Geometry check sheet. Reference: drawing and pictorial views, mm from the part's lowest x, y, z. Give positions to 0.01 mm unless a question says otherwise; leave off trailing zeros. Write each loop counter-clockwise with the first axis right and the second up, starting at its lowest first coordinate (ties: lowest second). Pieces come first, ordered by that corner, then holes. Notation, with made-up numbers: (-14.75, 6.25) -> (25.25, 6.25) arc R21 cw to (25.25, 40.25) -> close; hole circle Ø2 at (-24, 80.25). An arc over 180 degrees is marked (long way). Use a Markdown table: item, result. Add a question column.
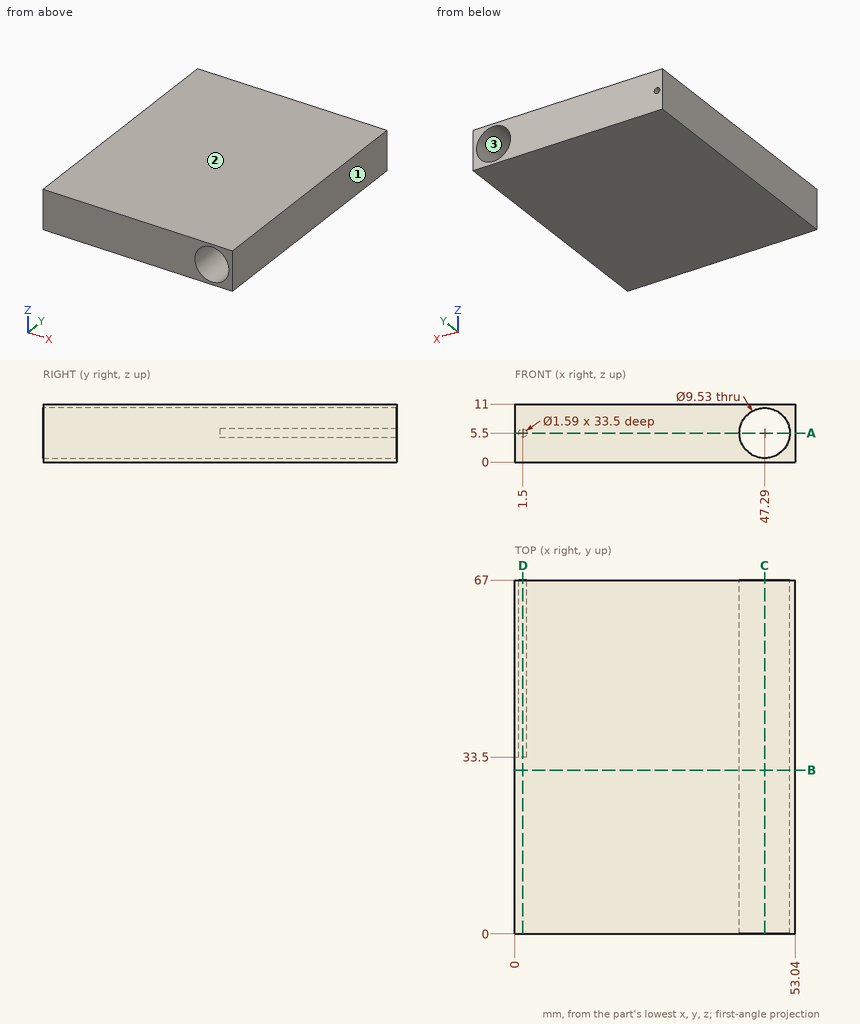
1) Draft check along X on the marked faces 1, 2 and 3. Enter one of: +X half, -X half, draft (parallel to the pull), parting line (faces both ways), or undercut.
2) Sectioned sample at C-C, the plane x = 47.29. Enter the section's corners in (y, z) (3 decimals).
3) Sectioned sample at A-A, the plane z = 5.5. Enter the section's corners in (x, y) (3 decimals).
4) Sectioned sample at D-D, the plane x = 1.5. Enter the section's corners in (y, z) (3 decimals), and give its area (3 significant figures).
5) Sectioned sample at B-B, the plane y = 31. Enter the section's corners in (x, z) (3 decimals).
6) Material ranges on probe 1 along X at (y, z) = (48, 5.5) (3 decimals); probe 2 along Z at (x, y) = (47, 23); probe 3 along X at (y, z) = (60, 6.5), recorded low to high. Write a range as [from, to].
7) Gauge pin test, flat ends, axial feed: P1, Ø5, axis at x = 36.5, z = 5, coming from the -Y side; P2, Ø1.4, axis at x = 1.5, z = 5.5, coming from the +Y side. Record the tip position at first contact, or that the pin passes through.
Check values:
| question | item | result |
|---|---|---|
| 1 | face 1 | +X half |
| 1 | face 2 | draft |
| 1 | face 3 | undercut |
| 2 | outline | (0, 0) -> (67, 0) -> (67, 0.735) -> (0, 0.735) -> close; (0, 10.265) -> (67, 10.265) -> (67, 11) -> (0, 11) -> close |
| 3 | outline | (0, 0) -> (42.525, 0) -> (42.525, 67) -> (2.295, 67) -> (2.295, 33.5) -> (0.705, 33.5) -> (0.705, 67) -> (0, 67) -> close; (52.055, 0) -> (53.04, 0) -> (53.04, 67) -> (52.055, 67) -> close |
| 4 | outline | (0, 0) -> (67, 0) -> (67, 4.705) -> (33.5, 4.705) -> (33.5, 6.295) -> (67, 6.295) -> (67, 11) -> (0, 11) -> close |
| 4 | area | 684 mm² |
| 5 | outline | (0, 0) -> (53.04, 0) -> (53.04, 11) -> (0, 11) -> close; hole circle Ø9.53 at (47.29, 5.5) |
| 6 | probe 1 | [0, 0.705], [2.295, 42.525], [52.055, 53.04] |
| 6 | probe 2 | [0, 0.74], [10.26, 11] |
| 6 | probe 3 | [0, 42.63], [51.95, 53.04] |
| 7 | P1 | y = 0 |
| 7 | P2 | y = 33.5 |
